from build123d import *

# Parameters (mm, degrees)
F0_W      = 30
F0_H      = 75
F1_DEPTH  = 30
F4_DEPTH  = 30.001
F2_W      = 30
F2_H      = 5.5
F5_DEPTH  = 25
F3_R      = 3.45
F6_DEPTH  = 30.001
F7_W      = 4.8
F7_H      = 30
F8_DEPTH  = 25
F10_DEPTH = 22.801
F9_R      = 3.45
F11_DEPTH = 22.801


with BuildPart() as f1:
    # F0 (on Right) → F1 (new body)
    with BuildSketch(Plane.YZ):
        Rectangle(F0_W, F0_H)
    extrude(amount=F1_DEPTH)

    # F3 (on face) → F4 (cut, through all)
    with BuildSketch(Plane(origin=(0, 15, 0), x_dir=(-1, 0, 0), z_dir=(0, 1, 0))):
        with BuildLine():
            ThreePointArc((-15, -37.5), (-25.6066017178, -33.1066017178), (-30, -22.5))
            Line((-30, -22.5), (-30, -37.5))
            Line((-30, -37.5), (-15, -37.5))
        make_face()
        with BuildLine():
            ThreePointArc((0, -22.5), (-4.3933982822, -33.1066017178), (-15, -37.5))
            Line((-15, -37.5), (0, -37.5))
            Line((0, -37.5), (0, -22.5))
        make_face()
    extrude(amount=-F4_DEPTH, mode=Mode.SUBTRACT)

    # F2 (on face) → F5 (cut)
    with BuildSketch(Plane(origin=(0, 0, -37.5), x_dir=(1, 0, 0), z_dir=(0, 0, -1))):
        with Locations((15, 5.25)):
            Rectangle(F2_W, F2_H)
        with Locations((15, -5.25)):
            Rectangle(F2_W, F2_H)
    extrude(amount=-F5_DEPTH, mode=Mode.SUBTRACT)

    # F3 (on face) → F6 (cut, through all)
    with BuildSketch(Plane(origin=(0, 15, 0), x_dir=(-1, 0, 0), z_dir=(0, 1, 0))):
        with Locations((-15, -22.5)):
            Circle(F3_R)
    extrude(amount=-F6_DEPTH, mode=Mode.SUBTRACT)

    # F7 (on face) → F8 (join)
    with BuildSketch(Plane.XY.offset(37.5)):
        with Locations((9.6, 0)):
            Rectangle(F7_W, F7_H)
        with Locations((20.4, 0)):
            Rectangle(F7_W, F7_H)
    extrude(amount=F8_DEPTH)

    # F9 (on face) → F10 (cut, through all)
    with BuildSketch(Plane(origin=(7.2, 0, 0), x_dir=(0, -1, 0), z_dir=(-1, 0, 0))):
        with BuildLine():
            ThreePointArc((-15, 50.5), (-9.6046863561, 59.1308579452), (0, 62.5))
            Line((0, 62.5), (-15, 62.5))
            Line((-15, 62.5), (-15, 50.5))
        make_face()
        with BuildLine():
            ThreePointArc((0, 62.5), (9.6046863561, 59.1308579452), (15, 50.5))
            Line((15, 50.5), (15, 62.5))
            Line((15, 62.5), (0, 62.5))
        make_face()
    extrude(amount=-F10_DEPTH, mode=Mode.SUBTRACT)

    # F9 (on face) → F11 (cut, through all)
    with BuildSketch(Plane(origin=(7.2, 0, 0), x_dir=(0, -1, 0), z_dir=(-1, 0, 0))):
        with Locations((0, 50.5)):
            Circle(F9_R)
    extrude(amount=-F11_DEPTH, mode=Mode.SUBTRACT)


solid = f1.part
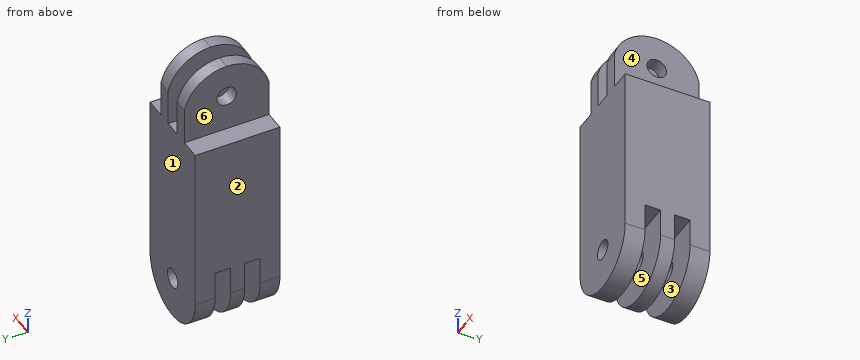
The model under review builds one solid part; all positions refer to its coordinate system, in mm. Face numbers are marked on the shaded views. A direction names the side the tool comes from. Coordinates: 2 decimals unless noted, no trailing zeros. Loops run counter-clockwise (first coordinate to the right, second up) from the corner with the lowest first, then second, coordinate; pieces in that order, holes last. Notation, with made-up numbers: M 7.5,24.5 L 48.5,24.5 A25 ccw 48.5,45.5 Z; hole C -31,38.5 d6. An arc over 180 degrees is marked long. Put each result on its own line as item: value. Start each with the question number.
Q1. Add section D-D (x = 3.5). Write out the cut boundary in (y, z), and give its area (3 significant figures).
Q2. Wall thickness on line 1 (Y direction, x = 2.75, z = -30); line 2 (Z direction, x = 15, y = 1.2); line 3 (Y direction, x = 19.75, z = 51): over which ranges is each line inside the solid? List them lowest first.
Q3. The part is to be moulded in two halves that separate along Y. For the marked faces 1, 2 and 3, say which applies: +Y half, -Y half, draft (parallel to the pull), parting line (faces both ways), or undercut.
Q4. Clearance check with flat-ended pins moving along their axes: pin 1 (6 mm diameter, centred on x = 27, y = 6.5, fed in from +Z); pin 2 (7.5 mm diameter, centred on y = -3, z = 51, fed in from -X); pin 3 (5 mm diameter, centred on x = 5, y = -11.5, fed in from -Z); pin 4 (4 mm diameter, centred on y = 0, z = 50.5, fed in from -X). State where each tip first meets the part, or that it passes through.
Q5. For the marked faces 4, 5 and 6, list the 3-axis set-ups (+Z, -Z, +X, -X, +Y, -Y) from which the entire face can be reached by the end or side of a thin tool; tool diameter is ignored.
Q6. Add section C-C (y = -7). Write out the cut boundary in (x, z).
Q7. Add section B-B (z = -25). Write out the cut boundary in (x, y).
Q8. Add section A-A (x = 15). Write out the cut boundary in (y, z).
Answers:
1. outline: M -15,-32.13 L -8,-32.13 L -8,-12.5 L -2.5,-12.5 L -2.5,-32.13 L 2.5,-32.13 L 2.5,-12.5 L 8,-12.5 L 8,-32.13 L 15,-32.13 L 15,37.5 L -15,37.5 Z
1. area: 1,870 mm^2
2. line 1: y = -15 to -8, -2.5 to 2.5, 8 to 15
2. line 2: z = -37.5 to -25.95, -19.05 to 37.5
2. line 3: y = -14.88 to -3.41, 3.41 to 14.88
3. face 1: +Y half
3. face 2: draft
3. face 3: undercut
4. pin 1: stops at z = 37.5
4. pin 2: stops at x = 7.2
4. pin 3: stops at z = -35.49
4. pin 4: passes through
5. face 4: +Z, +X, +Y, -Y
5. face 5: -Z, +X, -X
5. face 6: +Z, -X, +Y, -Y
6. outline: M 0,-12.5 L 30,-12.5 L 30,37.5 L 22.8,37.5 L 22.8,60.81 L 18,60.81 L 18,37.5 L 12,37.5 L 12,60.81 L 7.2,60.81 L 7.2,37.5 L 0,37.5 Z
7. outline: M 0.21,-15 L 12.62,-15 L 12.62,-8 L 0.21,-8 Z; M 0.21,-2.5 L 12.62,-2.5 L 12.62,2.5 L 0.21,2.5 Z; M 0.21,8 L 12.62,8 L 12.62,15 L 0.21,15 Z; M 17.38,-15 L 29.79,-15 L 29.79,-8 L 17.38,-8 Z; M 17.38,-2.5 L 29.79,-2.5 L 29.79,2.5 L 17.38,2.5 Z; M 17.38,8 L 29.79,8 L 29.79,15 L 17.38,15 Z
8. outline: M -15,-37.5 L -8,-37.5 L -8,-25.95 L -15,-25.95 Z; M -15,-19.05 L -8,-19.05 L -8,-12.5 L -2.5,-12.5 L -2.5,-19.05 L 2.5,-19.05 L 2.5,-12.5 L 8,-12.5 L 8,-19.05 L 15,-19.05 L 15,37.5 L -15,37.5 Z; M -2.5,-37.5 L 2.5,-37.5 L 2.5,-25.95 L -2.5,-25.95 Z; M 8,-37.5 L 15,-37.5 L 15,-25.95 L 8,-25.95 Z
